Can you work these out from the model? Positions are in its coordinate system, mm. Face numbers are marked on the shaded views. A direction names the side the tool comes from. Round coordinates to 2 decimals unless told otherwise and drop trailing zeros. Write each loop counter-clockwise with the first axis right and the second up, starting at its lowest first coordinate (ties: lowest second). Pieces come first, ordered by that corner, then holes. Notation, with made-up numbers: (17.5, 63) - (55.5, 63) arc R25 cw to (55.5, 98) - close; hole circle Ø5 at (67.5, 32.25). An arc over 180 degrees is marked (long way). One line per item, written item: value. Start each with the question number.
(1) I want a section at C-C on x = -26. List the corners of the cut face in (y, z) for me, plus the area to 3 significant figures.
(2) I want a section at B-B on z = 5.25. List the corners of the cut face in (x, y) for me, plus the area to 3 significant figures.
(3) On a 3-axis mill with a long thin cutter (end or side, diameter ignored), from which of +Z, -Z, +X, -X, +Y, -Y can I reach the whole of each face in a straight line? I mean the marked faces 4, 5 and 6. Say none if no direction works.
(4) If I drill on L1, parallel to Y at x = -25, z = 20; L2, parallel to X at y = -4, z = 10; L3, parallel to Z at x = 2.5, y = 10.5, over which ranges is the centre line in solid material (lowest first)? Write a range as from..to.
(5) I want a section at D-D on z = 20. List the corners of the cut face in (x, y) for me.
(6) I want a section at A-A on y = -23.5. List the corners of the cut face in (x, z) for me.
(7) I'm going to push flat-ended pins straight in: pin 1 Ø2 at (x, y) = (4, 7) entering from +Z; pin 2 Ø2.5 at (x, z) = (-15, 1.5) entering from -Y; pin 3 Ø3 at (x, y) = (-28, -35.5) entering from -Z. Where does each tip first touch, or does it pass through?
(8) Thinking about a two-plate mould opening in X: for the marked faces 1, 2 and 3, which applies, +X half, -X half, draft (parallel to the pull), parting line (faces both ways), or undercut?
Autodesk Inventor part; units mm, degrees
ref_plane "YZ Plane" through (0, 0, 0) normal (1, 0, 0) x (0, 1, 0)
ref_plane "XZ Plane" through (0, 0, 0) normal (0, 1, 0) x (-1, 0, 0)
ref_plane "XY Plane" through (0, 0, 0) normal (0, 0, 1) x (1, 0, 0)
sketch "スケッチ1" plane through (0, 0, 0) normal (0, 0, 1) x (1, 0, 0)
  line L0 (-32.5, 15) -> (32.5, 15)
  line L1 (32.5, 15) -> (32.5, -15)
  line L2 (32.5, -15) -> (-32.5, -15)
  line L3 (-32.5, -15) -> (-32.5, 15)
  line L4 (-45.5, 0) -> (45.5, 0)
  line L5 (0, 21) -> (0, -21)
  point P0 (0, 0)
  dimension "d0" = 30
  dimension "d1" = 65
extrude "押し出し1" add sketch "スケッチ1" along normal blind 3
sketch "スケッチ2" plane through (0, 0, 3) normal (0, 0, 1) x (1, 0, 0)
  line L0 (32.5, 15) -> (-32.5, 15)
  line L1 (-32.5, 15) -> (-22.5, 15)
  line L2 (-22.5, 15) -> (-22.5, -45)
  line L3 (-22.5, -45) -> (-32.5, -45)
  line L4 (-32.5, -45) -> (-32.5, 15)
  line L5 (32.5, -15) -> (32.5, 15)
  line L6 (32.5, 15) -> (22.5, 15)
  line L7 (22.5, 15) -> (22.5, -45)
  line L8 (22.5, -45) -> (32.5, -45)
  line L9 (32.5, -45) -> (32.5, 15)
  point P0 (0, 0)
  dimension "d4" = 60
  dimension "d5" = 10
extrude "押し出し2" add sketch "スケッチ2" along normal blind 21
sketch "スケッチ3" plane through (32.5, -15, 0) normal (1, 0, 0) x (0, 0, -1)
  circle A0 centre (-20, -25) radius 3
  line L0 (-24, -30) -> (-24, 30)
  line L1 (-3, -30) -> (-24, -30)
  point P0 (0, 15)
  dimension "d8" = 4
  dimension "d9" = 5
  dimension "d10" = 6
extrude "押し出し3" cut sketch "スケッチ3" against normal up to surface (65 mm away)
properties part number "vacuum_cup_base"
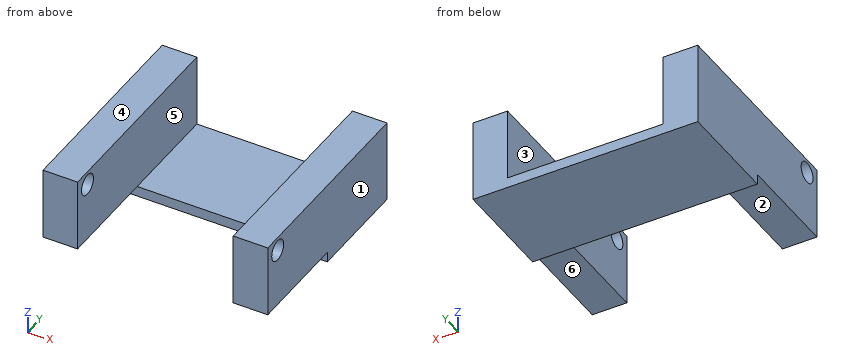
Established:
1. outline: (-45, 3) - (-15, 3) - (-15, 0) - (15, 0) - (15, 24) - (-45, 24) - close; hole circle Ø6 at (-40, 20)
1. area: 1,320 mm2
2. outline: (-32.5, -45) - (-22.5, -45) - (-22.5, 15) - (-32.5, 15) - close; (22.5, -45) - (32.5, -45) - (32.5, 15) - (22.5, 15) - close
2. area: 1,200 mm2
3. face 4: +Z, +X, -X, +Y, -Y
3. face 5: +Z, +Y, -Y
3. face 6: -Z, +X, -X, -Y
4. L1: -45..-43, -37..15
4. L2: -32.5..-22.5, 22.5..32.5
4. L3: 0..3
5. outline: (-32.5, -45) - (-22.5, -45) - (-22.5, -43) - (-32.5, -43) - close; (-32.5, -37) - (-22.5, -37) - (-22.5, 15) - (-32.5, 15) - close; (22.5, -45) - (32.5, -45) - (32.5, -43) - (22.5, -43) - close; (22.5, -37) - (32.5, -37) - (32.5, 15) - (22.5, 15) - close
6. outline: (-32.5, 3) - (-22.5, 3) - (-22.5, 24) - (-32.5, 24) - close; (22.5, 3) - (32.5, 3) - (32.5, 24) - (22.5, 24) - close
7. pin 1: z = 3
7. pin 2: y = -15
7. pin 3: z = 3
8. face 1: +X half
8. face 2: draft
8. face 3: undercut
